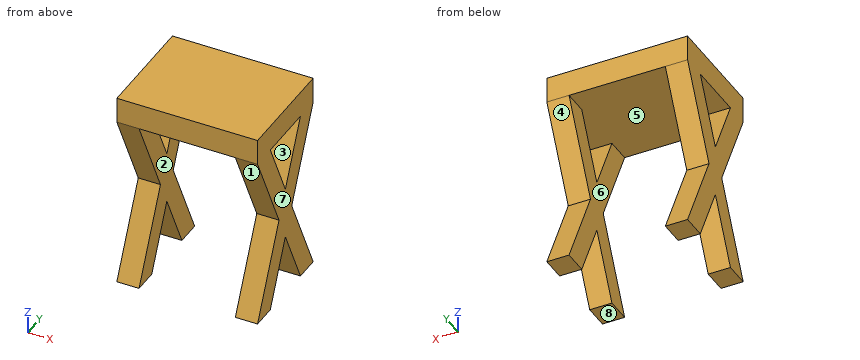
```python
from build123d import *

# Parameters (mm, degrees)
F0_W     = 482.6
F0_H     = 368.3
F1_DEPTH = 88.9
F3_DEPTH = 482.6
F4_W     = 330.2
F4_H     = 596.9
F5_DEPTH = 368.301


with BuildPart() as f1:
    # F0 (on Top) → F1 (new body)
    with BuildSketch(Plane.XY):
        Rectangle(F0_W, F0_H)
    extrude(amount=F1_DEPTH)

    # F2 (on face) → F3 (join)
    with BuildSketch(Plane.YZ.offset(241.3)):
        Polygon((-99.7690824552, 0), (-184.15, 0), (-42.1904587724, -298.45), (0, -209.7504852528), align=None)
        Polygon((99.7690824552, 0), (0, -209.7504852528), (42.1904587724, -298.45), (184.15, 0), align=None)
        Polygon((0, -209.7504852528), (-42.1904587724, -298.45), (0, -387.1495147472), (42.1904587724, -298.45), align=None)
        Polygon((42.1904587724, -298.45), (0, -387.1495147472), (99.7690824552, -596.9), (184.15, -596.9), align=None)
        Polygon((0, -387.1495147472), (-42.1904587724, -298.45), (-184.15, -596.9), (-99.7690824552, -596.9), align=None)
    extrude(amount=-F3_DEPTH)

    # F4 (on face) → F5 (cut, through all)
    with BuildSketch(Plane(origin=(0, 184.15, 0), x_dir=(-1, 0, 0), z_dir=(0, 1, 0))):
        with Locations((0, -298.45)):
            Rectangle(F4_W, F4_H)
    extrude(amount=-F5_DEPTH, mode=Mode.SUBTRACT)


solid = f1.part
```
Verification items for the finished model (mm, model axes). Face numbers are marked on the shaded views. A direction names the side the tool comes from. Coordinates: 2 decimals unless noted, no trailing zeros. Order: outer loops, then holes, each group sorted by start corner. A loop starts at its lowest first (then second) coordinate and runs counter-clockwise, first axis right, second up. Notation, with made-up numbers: (87, 11.25) -> (142, 11.25) arc R17 ccw to (142, 36.25) -> close; hole circle Ø2 at (-27, -28). An arc over 180 degrees is marked (long way). Answer as CSV lines item,"result". Start each with the question number.
1) Gauge pin test, flat ends, axial feed: pin 1 Ø12 at (y, z) = (102, -181) entering from +X; pin 2 Ø10 at (x, z) = (161.5, -354.5) entering from -Y. Record the tip position at first contact, or that the pin passes through.
2) Set-up check for the marked faces 1, 2, 3, 4 and 5: record each of +Z, -Z, +X, -X, +Y, -Y from which the full face is reachable in a straight line by a thin tool's end or side.
3) Release check for a two-part mould opening along X. For the marked faces 6, 7 and 8 record: released by +X, released by -X, zero draft, split by the parting line, or undercut.
4) Cross-section at D-D, the plane z = -148.5. Record the boundary of the cut face in (x, y), then the cut area to 3 significant figures.
5) Cross-section at A-A, the plane y = -13. Record the boundary of the cut face in (x, z).
6) Material ranges on L1, parallel to X at y = -109, z = -101; L2, parallel to Z at x = -23, y = -7; L3, parallel to Z at x = 192, y = 65, recorded low to high. Write a range as [from, to].
7) Cross-section at C-C, the plane z = -285. Record the boundary of the cut face in (x, y).
8) Cross-section at B-B, the plane x = 176. Record the boundary of the cut face in (y, z), then the cut area to 3 significant figures.
Conclusion:
1,pin 1,"stops at x = 241.3"
1,pin 2,"stops at y = -70.5"
2,face 1,"+X, -X, -Y"
2,face 2,"-Z, +Y, -Y"
2,face 3,"+X, -X"
2,face 4,"+X, -X, +Y"
2,face 5,"none"
3,face 6,"undercut"
3,face 7,"released by +X"
3,face 8,"zero draft"
4,outline,"(-241.3, -113.52) -> (-165.1, -113.52) -> (-165.1, -29.13) -> (-241.3, -29.13) -> close; (-241.3, 29.13) -> (-165.1, 29.13) -> (-165.1, 113.52) -> (-241.3, 113.52) -> close; (165.1, -113.52) -> (241.3, -113.52) -> (241.3, -29.13) -> (165.1, -29.13) -> close; (165.1, 29.13) -> (241.3, 29.13) -> (241.3, 113.52) -> (165.1, 113.52) -> close"
4,area,"25,700 mm²"
5,outline,"(-241.3, -414.48) -> (-165.1, -414.48) -> (-165.1, -182.42) -> (-241.3, -182.42) -> close; (-241.3, 0) -> (241.3, 0) -> (241.3, 88.9) -> (-241.3, 88.9) -> close; (165.1, -414.48) -> (241.3, -414.48) -> (241.3, -182.42) -> (165.1, -182.42) -> close"
6,L1,"x = [-241.3, -165.1], [165.1, 241.3]"
6,L2,"z = [0, 88.9]"
6,L3,"z = [-523.8, -346.4], [-250.5, -73.1], [0, 88.9]"
7,outline,"(-241.3, -48.59) -> (-165.1, -48.59) -> (-165.1, 48.59) -> (-241.3, 48.59) -> close; (165.1, -48.59) -> (241.3, -48.59) -> (241.3, 48.59) -> (165.1, 48.59) -> close"
8,outline,"(-184.15, -596.9) -> (-99.77, -596.9) -> (0, -387.15) -> (99.77, -596.9) -> (184.15, -596.9) -> (42.19, -298.45) -> (184.15, 0) -> (184.15, 88.9) -> (-184.15, 88.9) -> (-184.15, 0) -> (-42.19, -298.45) -> close; hole (-99.77, 0) -> (0, -209.75) -> (99.77, 0) -> close"
8,area,"126,000 mm²"
